Source: CAD feature listing. Evaluate the final solid. Frame: model axes, mm. A direction names the side the tool comes from. Round coordinates to 2 decimals unless told otherwise and drop trailing zeros. Loops run counter-clockwise (first coordinate to the right, second up) from the corner with the lowest first, then second, coordinate; pieces in that order, holes last.
Item 1: Section query C-C on y = 5.5. Return loops of the section in (x, z), then the cut area to 3 significant figures.
Item 2: Section query A-A on z = 29. Return loops of the section in (x, y).
Item 3: Access query for faces 1 (the flat face through (26, 0.269, 20)), 2 (the cylindrical face through (10.11, 5.57, 30.25)), 3 (the flat face through (-7.634, 4, 20)), 4 (the flat face through (-5, 0.269, 20)). Directions: +Z, -Z, +X, -X, +Y, -Y. A direction counts if a zero-diameter tool reaches every point of the face in a straight line with its end or side. Return the directions, or none.
Item 4: Pull-direction query (Y, two-part tool) for faces 5 (the flat face through (26, -3.131, 20)), 6 (the flat face through (11, 10.269, 20)), 7 (the flat face through (10, -2, 40)); classes: released by +Y, released by -Y, zero draft, split by the parting line, or undercut.
Item 5: Ray query, L1, parallel to Y at x = 7, z = 18; L2, parallel to Y at x = 22.5, z = 16; L3, parallel to X at y = -1.25, z = 38.5. Return the intervals inside material, ascending.
Item 6: Section query D-D on z = 7. Return loops of the section in (x, y).
Item 7: Section query B-B on x = 8. Return loops of the section in (y, z), then the cut area to 3 significant figures.
Item 8: First-contact query: P1, Ø2.5, axis at x = 26.5, z = 11.5, coming from the -Y side; P2, Ø3, axis at y = -11.5, z = 9, coming from the +X side; P3, Ø4, axis at y = -6, z = 28, coming from the +X side. Flat tips, straight axial feed; report the tip coordinate or a pass-through.
```python
from build123d import *

# Parameters (mm, degrees)
BOSS_EXTRUDE3_DEPTH = 40
CUT_EXTRUDE1_DEPTH  = 72


# Read off the part's stored shape, not the designer's step: Boss-Extrude3
with BuildPart() as part:
    # Boss-Extrude3 outline → Boss-Extrude3 (new body)
    with BuildSketch(Plane.XY):
        with BuildLine():
            Line((28.365517241, -3.131034483), (23.165517241, -3.131034483))
            ThreePointArc((23.165517241, -3.131034483), (21.465517241, -1.431034483), (23.165517241, 0.268965517))
            Line((23.165517241, 0.268965517), (28.365517241, 0.268965517))
            Line((28.365517241, 0.268965517), (28.365517241, 10.268965517))
            Line((28.365517241, 10.268965517), (-7.634482759, 10.268965517))
            Line((-7.634482759, 10.268965517), (-7.634482759, 0.268965517))
            Line((-7.634482759, 0.268965517), (-1.734482759, 0.268965517))
            ThreePointArc((-1.734482759, 0.268965517), (-0.384482759, -1.781034483), (-2.434482759, -3.131034483))
            Line((-2.434482759, -3.131034483), (-7.634482759, -3.131034483))
            Line((-7.634482759, -3.131034483), (1.493101299, -14.008865575))
            Line((1.493101299, -14.008865575), (19.237933184, -14.008865575))
            Line((19.237933184, -14.008865575), (28.365517241, -3.131034483))
        make_face()
    extrude(amount=BOSS_EXTRUDE3_DEPTH)

    # Sketch4 → Cut-Extrude1 (cut)
    with BuildSketch(Plane.ZY.offset(7.634482759)):
        with BuildLine():
            Line((10.45, 6.251111401), (29.55, 6.251111401))
            ThreePointArc((29.55, 6.251111401), (30.25, 5.551111401), (29.55, 4.851111401))
            Line((29.55, 4.851111401), (10.45, 4.851111401))
            ThreePointArc((10.45, 4.851111401), (9.75, 5.551111401), (10.45, 6.251111401))
        make_face()
    extrude(amount=-CUT_EXTRUDE1_DEPTH, mode=Mode.SUBTRACT)


solid = part.part
```
Data:
1. outline: (-7.63, 0) - (28.37, 0) - (28.37, 9.75) - (-7.63, 9.75) - close; (-7.63, 30.25) - (28.37, 30.25) - (28.37, 40) - (-7.63, 40) - close
1. area: 702 mm2
2. outline: (-7.63, -3.13) - (1.49, -14.01) - (19.24, -14.01) - (28.37, -3.13) - (23.17, -3.13) arc R1.7 cw to (23.17, 0.27) - (28.37, 0.27) - (28.37, 4.85) - (-7.63, 4.85) - (-7.63, 0.27) - (-1.73, 0.27) arc R1.74 cw to (-2.43, -3.13) - close; (-7.63, 6.25) - (28.37, 6.25) - (28.37, 10.27) - (-7.63, 10.27) - close
3. face 1: +Z, -Z, +X
3. face 2: +X, -X
3. face 3: +Z, -Z, -X, +Y, -Y
3. face 4: +Z, -Z, -X
4. face 5: undercut
4. face 6: released by +Y
4. face 7: zero draft
5. L1: y = -14.01 to 4.85, 6.25 to 10.27
5. L2: y = -10.12 to -3, 0.13 to 4.85, 6.25 to 10.27
5. L3: x = -0.36 to 21.48
6. outline: (-7.63, -3.13) - (1.49, -14.01) - (19.24, -14.01) - (28.37, -3.13) - (23.17, -3.13) arc R1.7 cw to (23.17, 0.27) - (28.37, 0.27) - (28.37, 10.27) - (-7.63, 10.27) - (-7.63, 0.27) - (-1.73, 0.27) arc R1.74 cw to (-2.43, -3.13) - close
7. outline: (-14.01, 0) - (10.27, 0) - (10.27, 40) - (-14.01, 40) - close; hole (4.85, 10.45) arc R0.7 ccw to (6.25, 10.45) - (6.25, 29.55) arc R0.7 ccw to (4.85, 29.55) - close
7. area: 943 mm2
8. P1: stops at y = -6.84
8. P2: stops at x = 22.6
8. P3: stops at x = 27.64
